Read the model definition and answer for the solid it produces. Units are mm, in the model's axes. A direction names the side the tool comes from. Round coordinates to 2 decimals unless told otherwise and drop trailing zeros. Loops run counter-clockwise (first coordinate to the right, second up) from the corner with the lowest first, then second, coordinate; pieces in that order, holes last. Notation, with made-up numbers: M 58,57 L 73,57 A30 ccw 73,89 Z; hole C 75,3 d8. An arc over 180 degrees is marked long. Write each question's results on one line, items separated by ' | '.
Autodesk Inventor part; units mm, degrees
ref_plane "YZ Plane" through (0, 0, 0) normal (1, 0, 0) x (0, 1, 0)
ref_plane "XZ Plane" through (0, 0, 0) normal (0, 1, 0) x (-1, 0, 0)
sketch "Boceto1" plane through (0, 0, 0) normal (0, 1, 0) x (-1, 0, 0)
  circle A0 centre (0, 0) radius 12.5
  dimension "d0" = 25
extrude "Extrusión1" add sketch "Boceto1" along normal blind 30
sketch "Boceto2" plane through (0, 0, 0) normal (0, -1, 0) x (1, 0, 0)
  circle A0 centre (0, 0) radius 8
  dimension "d3" = 16
extrude "Extrusión2" cut sketch "Boceto2" against normal through all
sketch "Boceto3" plane through (0, 30, 0) normal (0, 1, 0) x (1, 0, 0)
  line L0 (6, 10.3923) -> (12, 0)
  line L1 (12, 0) -> (6, -10.3923)
  line L2 (6, -10.3923) -> (-6, -10.3923)
  line L3 (-6, -10.3923) -> (-12, 0)
  line L4 (-12, 0) -> (-6, 10.3923)
  line L5 (-6, 10.3923) -> (6, 10.3923)
  point P0 (0, 0)
  point P1 (0, 0)
  point P2 (0, 10.3923)
  dimension "d6" = 12
extrude "Extrusión3" cut sketch "Boceto3" against normal blind 4
sketch "Boceto4" plane through (0, 0, 0) normal (0, -1, 0) x (1, 0, 0)
  circle A0 centre (0, 0) radius 12.5
  arc A1 (30.0364, -5.1409) -> (30.0797, 4.8584) centre (29.9997, -0.141) ccw
  line L0 (30.0364, -5.1409) -> (3.1308, -12.1016)
  circle A2 centre (0, 0) radius 12.5
  line L1 (30.0797, 4.8584) -> (3.2448, 12.0715)
  dimension "d9" = 10
  dimension "d10" = 30
extrude "Extrusión4" add sketch "Boceto4" against normal blind 4 contours A0 L1 A1 L0
sketch "Boceto5" plane through (0, 30, 0) normal (0, 1, 0) x (1, 0, 0)
  arc A0 (-30, 5) -> (-30, -5) centre (-30, 0) ccw
  line L0 (-30, -5) -> (-3.1942, -12.085)
  circle A1 centre (0, 0) radius 12.5
  line L1 (-30, 5) -> (-3.1942, 12.085)
  dimension "d13" = 10
  dimension "d14" = 30
extrude "Extrusión5" add sketch "Boceto5" against normal blind 4 contours L1 A1 L0 A0
hole "Agujero1" at (29.9997, 4, -0.141) direction (0, -1, 0) diameter 4 depth 8 tip angle 118
hole "Agujero2" at (-30, 30, 0) direction (0, -1, 0) diameter 3 depth 8 tip angle 118
properties part number "steering_stand_off" material "Goma"
Item 1: The mould has two halves that part along Z. Classify faces 1 (the face through (-1.73, 12.82, -7.81)), 2 (the face through (16.9, 2, 8.4)), 3 (the face through (31.952, 1.972, -0.575)), 4 (the face through (-35, 28, 0)): pulls with the +Z half, pulls with the -Z half, needs draft (parallel to the pull), parting line crosses it, or undercut.
Outcome:
face 1: undercut | face 2: pulls with the +Z half | face 3: undercut | face 4: parting line crosses it
Item 2: The part is cut by section A-A (x = 0). Determine the outline of the cut face in (y, z), plus the area to 3 significant figures.
Outcome:
outline: M 0,-12.5 L 30,-12.5 L 30,-10.39 L 26,-10.39 L 26,-8 L 0,-8 Z; M 0,8 L 26,8 L 26,10.39 L 30,10.39 L 30,12.5 L 0,12.5 Z | area: 251 mm2
Item 3: For faces 5 (the face through (12.488, 14.79, -0.55)), 6 (the face through (16.772, 1.972, -8.573)), 7 (the face through (0, 28, -10.392)), determine the directions among +Z, -Z, +X, -X, +Y, -Y from which every point of the face is accessible in a straight line to the end or side of a thin tool.
Outcome:
face 5: none | face 6: -Z, +X, +Y, -Y | face 7: +Y
Item 4: The part is cut by section B-B (z = 3). Determine the outline of the cut face in (x, y).
Outcome:
outline: M -34,26 L -12.13,26 L -12.13,0 L -7.42,0 L -7.42,26 L -10.27,26 L -10.27,30 L -34,30 Z; M 7.42,0 L 33.89,0 L 33.89,4 L 12.13,4 L 12.13,30 L 10.27,30 L 10.27,26 L 7.42,26 Z
Item 5: The part is cut by section C-C (y = 13.5). Determine the outline of the cut face in (x, z), plus the area to 3 significant figures.
Outcome:
outline: C 0,0 d25; hole C 0,0 d16 | area: 290 mm2
Item 6: The part is cut by section D-D (z = -9). Determine the outline of the cut face in (x, y), plus the area to 3 significant figures.
Outcome:
outline: M -14.87,26 L -8.67,26 L -8.67,0 L 15.12,0 L 15.12,4 L 8.67,4 L 8.67,30 L 6.8,30 L 6.8,26 L -6.8,26 L -6.8,30 L -14.87,30 Z | area: 517 mm2
Item 7: Flat-ended cylindrical pins translate along their axes: pin 1 (3 mm diameter, centred on y = 18, z = 3.5, fed in from +X); pin 2 (10 mm diameter, centred on x = 15.5, y = 25, fed in from +Z); pin 3 (1 mm diameter, centred on x = -12, y = 14.5, fed in from +Z). Find the tip coordinate at first contact, or state that the pin passes through.
Outcome:
pin 1: stops at x = 12.34 | pin 2: stops at z = 6.78 | pin 3: stops at z = 4.9
Item 8: Straight lines are drawn through the part: line 1 (X direction, y = 29.15, z = 0); line 2 (Z direction, x = -30, y = 27.4); line 3 (Z direction, x = -10, y = 27). For each, find the intervals that lie inside material, in ascending order.
Outcome:
line 1: x = -35 to -31.5, -28.5 to -12, 12 to 12.5 | line 2: z = -5 to -1.5, 1.5 to 5 | line 3: z = -10.29 to -3.46, 3.46 to 10.29
